from build123d import *

# Parameters (mm, degrees)
BOSS_EXTRU_1_DEPTH       = 15
ESQUISSE6_W              = 100
ESQUISSE6_H              = 15
ENL_V_MAT_EXTRU_1_DEPTH  = 215
ENL_V_MAT_EXTRU_10_REACH = 393.106
ESQUISSE11_R             = 2.25
ENL_V_MAT_EXTRU_11_REACH = 393.106
ESQUISSE8_R              = 2.25
CONG_10_R                = 10
CONG_11_R                = 2
ENL_V_MAT_EXTRU_12_REACH = 391.991


with BuildPart() as part:
    # Esquisse1 → Boss.-Extru.1 (new body)
    with BuildSketch(Plane(origin=(0, 0, 0), x_dir=(1, 0, 0), z_dir=(0, 1, 0))):
        Polygon((-76.643189126, -51.401333399), (63.356810874, 43.598666601), (163.356810874, 43.598666601), (303.356810874, -51.401333399), (303.356810874, -151.401333399), (163.356810874, -246.401333399), (63.356810874, -246.401333399), (-76.643189126, -151.401333399), align=None)
    extrude(amount=BOSS_EXTRU_1_DEPTH)

    # Esquisse6 → Enlèv. mat.-Extru.1 (cut)
    with BuildSketch(Plane.XY.offset(246.401333399)):
        with Locations((113.356810874, 7.5)):
            Rectangle(ESQUISSE6_W, ESQUISSE6_H)
    extrude(amount=-ENL_V_MAT_EXTRU_1_DEPTH, mode=Mode.SUBTRACT)

    # Esquisse11 → Enlèv. mat.-Extru.10 (cut, up to next)
    with BuildSketch(Plane(origin=(0, 15, 0), x_dir=(1, 0, 0), z_dir=(0, 1, 0)), mode=Mode.PRIVATE) as enl_v_mat_extru_10_sk1:
        with Locations(Location((53.356810874, -129.901333399, 0), (0, 0, 270))):
            Circle(ESQUISSE11_R)
    enl_v_mat_extru_10_tool1 = extrude(enl_v_mat_extru_10_sk1.sketch, amount=-ENL_V_MAT_EXTRU_10_REACH, mode=Mode.PRIVATE) & part.part
    # Esquisse11 → Enlèv. mat.-Extru.10 (cut, up to next)
    with BuildSketch(Plane(origin=(0, 15, 0), x_dir=(1, 0, 0), z_dir=(0, 1, 0)), mode=Mode.PRIVATE) as enl_v_mat_extru_10_sk2:
        with Locations(Location((53.356810874, -184.901333399, 0), (0, 0, 270))):
            Circle(ESQUISSE11_R)
    enl_v_mat_extru_10_tool2 = extrude(enl_v_mat_extru_10_sk2.sketch, amount=-ENL_V_MAT_EXTRU_10_REACH, mode=Mode.PRIVATE) & part.part
    # Esquisse11 → Enlèv. mat.-Extru.10 (cut, up to next)
    with BuildSketch(Plane(origin=(0, 15, 0), x_dir=(1, 0, 0), z_dir=(0, 1, 0)), mode=Mode.PRIVATE) as enl_v_mat_extru_10_sk3:
        with Locations(Location((173.356810874, -129.901333399, 0), (0, 0, 270))):
            Circle(ESQUISSE11_R)
    enl_v_mat_extru_10_tool3 = extrude(enl_v_mat_extru_10_sk3.sketch, amount=-ENL_V_MAT_EXTRU_10_REACH, mode=Mode.PRIVATE) & part.part
    # Esquisse11 → Enlèv. mat.-Extru.10 (cut, up to next)
    with BuildSketch(Plane(origin=(0, 15, 0), x_dir=(1, 0, 0), z_dir=(0, 1, 0)), mode=Mode.PRIVATE) as enl_v_mat_extru_10_sk4:
        with Locations(Location((173.356810874, -184.901333399, 0), (0, 0, 270))):
            Circle(ESQUISSE11_R)
    enl_v_mat_extru_10_tool4 = extrude(enl_v_mat_extru_10_sk4.sketch, amount=-ENL_V_MAT_EXTRU_10_REACH, mode=Mode.PRIVATE) & part.part
    add(enl_v_mat_extru_10_tool1.solids().sort_by_distance((53.356811, 15, 129.901333))[0], mode=Mode.SUBTRACT)
    add(enl_v_mat_extru_10_tool2.solids().sort_by_distance((53.356811, 15, 184.901333))[0], mode=Mode.SUBTRACT)
    add(enl_v_mat_extru_10_tool3.solids().sort_by_distance((173.356811, 15, 129.901333))[0], mode=Mode.SUBTRACT)
    add(enl_v_mat_extru_10_tool4.solids().sort_by_distance((173.356811, 15, 184.901333))[0], mode=Mode.SUBTRACT)

    # Esquisse8 → Enlèv. mat.-Extru.11 (cut, up to next)
    with BuildSketch(Plane(origin=(0, 15, 0), x_dir=(1, 0, 0), z_dir=(0, 1, 0)), mode=Mode.PRIVATE) as enl_v_mat_extru_11_sk1:
        with Locations(Location((180.356810874, -120.901333399, 0), (0, 0, 270))):
            Circle(ESQUISSE8_R)
    enl_v_mat_extru_11_tool1 = extrude(enl_v_mat_extru_11_sk1.sketch, amount=-ENL_V_MAT_EXTRU_11_REACH, mode=Mode.PRIVATE) & part.part
    # Esquisse8 → Enlèv. mat.-Extru.11 (cut, up to next)
    with BuildSketch(Plane(origin=(0, 15, 0), x_dir=(1, 0, 0), z_dir=(0, 1, 0)), mode=Mode.PRIVATE) as enl_v_mat_extru_11_sk2:
        with Locations(Location((180.356810874, -81.901333399, 0), (0, 0, 270))):
            Circle(ESQUISSE8_R)
    enl_v_mat_extru_11_tool2 = extrude(enl_v_mat_extru_11_sk2.sketch, amount=-ENL_V_MAT_EXTRU_11_REACH, mode=Mode.PRIVATE) & part.part
    # Esquisse8 → Enlèv. mat.-Extru.11 (cut, up to next)
    with BuildSketch(Plane(origin=(0, 15, 0), x_dir=(1, 0, 0), z_dir=(0, 1, 0)), mode=Mode.PRIVATE) as enl_v_mat_extru_11_sk3:
        with Locations(Location((46.356810874, -120.901333399, 0), (0, 0, 270))):
            Circle(ESQUISSE8_R)
    enl_v_mat_extru_11_tool3 = extrude(enl_v_mat_extru_11_sk3.sketch, amount=-ENL_V_MAT_EXTRU_11_REACH, mode=Mode.PRIVATE) & part.part
    # Esquisse8 → Enlèv. mat.-Extru.11 (cut, up to next)
    with BuildSketch(Plane(origin=(0, 15, 0), x_dir=(1, 0, 0), z_dir=(0, 1, 0)), mode=Mode.PRIVATE) as enl_v_mat_extru_11_sk4:
        with Locations(Location((46.356810874, -81.901333399, 0), (0, 0, 270))):
            Circle(ESQUISSE8_R)
    enl_v_mat_extru_11_tool4 = extrude(enl_v_mat_extru_11_sk4.sketch, amount=-ENL_V_MAT_EXTRU_11_REACH, mode=Mode.PRIVATE) & part.part
    add(enl_v_mat_extru_11_tool1.solids().sort_by_distance((180.356811, 15, 120.901333))[0], mode=Mode.SUBTRACT)
    add(enl_v_mat_extru_11_tool2.solids().sort_by_distance((180.356811, 15, 81.901333))[0], mode=Mode.SUBTRACT)
    add(enl_v_mat_extru_11_tool3.solids().sort_by_distance((46.356811, 15, 120.901333))[0], mode=Mode.SUBTRACT)
    add(enl_v_mat_extru_11_tool4.solids().sort_by_distance((46.356811, 15, 81.901333))[0], mode=Mode.SUBTRACT)

    # Congé10
    cong_10_edges = [part.edges().sort_by_distance(p)[0] for p in [
        (-76.643189126, 7.5, 51.401333399),
        (63.356810874, 7.5, -43.598666601),
        (163.356810874, 7.5, -43.598666601),
        (303.356810874, 7.5, 51.401333399),
        (303.356810874, 7.5, 151.401333399),
        (-76.643189126, 7.5, 151.401333399),
        (63.356810874, 7.5, 31.401333399),
        (163.356810874, 7.5, 31.401333399),
    ]]
    fillet(cong_10_edges, radius=CONG_10_R)

    # Congé11
    cong_11_edges = [part.edges().sort_by_distance(p)[0] for p in [
        (163.356810874, 7.5, 246.401333399),
        (63.356810874, 7.5, 246.401333399),
    ]]
    fillet(cong_11_edges, radius=CONG_11_R)

    # Esquisse12 → Enlèv. mat.-Extru.12 (cut, up to next)
    with BuildSketch(Plane(origin=(0, 15, 0), x_dir=(1, 0, 0), z_dir=(0, 1, 0)), mode=Mode.PRIVATE) as enl_v_mat_extru_12_sk1:
        with BuildLine():
            Line((46.009256573, -55.538188752), (18.058498347, -78.315798735))
            ThreePointArc((18.058498347, -78.315798735), (14.643777091, -83.767882822), (15.256670784, -90.171780344))
            Line((15.256670784, -90.171780344), (27.943631129, -118.361875593))
            ThreePointArc((27.943631129, -118.361875593), (31.633138728, -122.655474578), (37.06267458, -124.257847507))
            Line((37.06267458, -124.257847507), (53.356810874, -124.257847507))
            ThreePointArc((53.356810874, -124.257847507), (57.183645198, -123.496642832), (60.427878686, -121.328915318))
            Line((60.427878686, -121.328915318), (63.356810874, -118.39998313))
            Line((63.356810874, -118.39998313), (63.356810874, -59.592280682))
            Line((63.356810874, -59.592280682), (59.121809419, -54.561118788))
            ThreePointArc((59.121809419, -54.561118788), (52.42687157, -53.188778562), (46.009256573, -55.538188752))
        make_face()
    enl_v_mat_extru_12_tool1 = extrude(enl_v_mat_extru_12_sk1.sketch, amount=-ENL_V_MAT_EXTRU_12_REACH, mode=Mode.PRIVATE) & part.part
    # Esquisse12 → Enlèv. mat.-Extru.12 (cut, up to next)
    with BuildSketch(Plane(origin=(0, 15, 0), x_dir=(1, 0, 0), z_dir=(0, 1, 0)), mode=Mode.PRIVATE) as enl_v_mat_extru_12_sk2:
        with BuildLine():
            Line((166.285743062, -121.328915318), (163.356810874, -118.39998313))
            Line((163.356810874, -118.39998313), (163.356810874, -73.642376596))
            Line((163.356810874, -73.642376596), (176.462200108, -67.250451181))
            ThreePointArc((176.462200108, -67.250451181), (187.921289626, -66.549583242), (196.519678004, -74.156794674))
            Line((196.519678004, -74.156794674), (206.924784537, -95.490424571))
            ThreePointArc((206.924784537, -95.490424571), (205.909865534, -114.856232791), (188.948903611, -124.257847507))
            Line((188.948903611, -124.257847507), (173.356810874, -124.257847507))
            ThreePointArc((173.356810874, -124.257847507), (169.529976551, -123.496642832), (166.285743062, -121.328915318))
        make_face()
    enl_v_mat_extru_12_tool2 = extrude(enl_v_mat_extru_12_sk2.sketch, amount=-ENL_V_MAT_EXTRU_12_REACH, mode=Mode.PRIVATE) & part.part
    add(enl_v_mat_extru_12_tool1.solids().sort_by_distance((43.070441, 15, 90.852572))[0], mode=Mode.SUBTRACT)
    add(enl_v_mat_extru_12_tool2.solids().sort_by_distance((183.873626, 15, 97.045657))[0], mode=Mode.SUBTRACT)


solid = part.part
Could you check a few things on this model? Use its own coordinates, in mm. A direction names the side the tool comes from. Round coordinates to 2 decimals unless told otherwise and drop trailing zeros. Write each loop counter-clockwise with the first axis right and the second up, starting at its lowest first coordinate (ties: lowest second). Pieces come first, ordered by that corner, then holes. Notation, with made-up numbers: (6.25, 69.5) -> (21.25, 69.5) arc R14 cw to (21.25, 87.5) -> close; hole circle Ø2 at (0.25, 9.25). An arc over 180 degrees is marked (long way). Use a Markdown table: item, result.
1. For pin 1 Ø6 at (x, y) = (248, 13.5) entering from -Z; pin 2 Ø7.5 at (y, z) = (5, 161) entering from +X; pin 3 Ø3.5 at (x, z) = (53.36, 184.9) entering from +Y; pin 4 Ø7.5 at (x, y) = (116.5, 6.5) entering from +Z, each with a flat end and sliding along its axis, tell me the tip position at first contact or that it passes through.
Answer key:
| item | result |
|---|---|
| pin 1 | stops at z = 11.8 |
| pin 2 | stops at x = 294.74 |
| pin 3 | passes through |
| pin 4 | stops at z = 31.4 |
2. If we section it at D-D (x = -36): List the corners of the cut face in (y, z) for me.
Answer key:
| item | result |
|---|---|
| outline | (0, 23.82) -> (15, 23.82) -> (15, 178.98) -> (0, 178.98) -> close |
3. Please list where these lines run through material, in increasing order: probe 1 along X at (y, z) = (12.5, 135); probe 2 along X at (y, z) = (8.25, 69); probe 3 along X at (y, z) = (1.75, 58.5).
Answer key:
| item | result |
|---|---|
| probe 1 | x = -76.64 to 63.36, 163.36 to 303.36 |
| probe 2 | x = -76.64 to 29.49, 163.36 to 172.88, 192.38 to 303.36 |
| probe 3 | x = -76.64 to 42.37, 62.44 to 63.36, 163.36 to 303.36 |
4. Which directions (+Z, -Z, +X, -X, +Y, -Y) give clear straight access to the entire face, cutting with the end or side of a thin tool? Please do faces 4 (the face through (187.77, 7.6, 66.5)), 5 (the face through (-76.643, 7, 102)), 6 (the face through (63.357, 7, 181)).
Answer key:
| item | result |
|---|---|
| face 4 | +Y, -Y |
| face 5 | +Z, -Z, -X, +Y, -Y |
| face 6 | +Z, +Y, -Y |
5. We'd pull the mould along Z, two halves only. Please class faces 1 (the face through (160.35, 7.605, 34.253)), 2 (the face through (113, 7, -43.599)), 3 (the face through (181, 8, 124.258)): +Z half, -Z half, draft (parallel to the pull), parting line (faces both ways), or undercut.
Answer key:
| item | result |
|---|---|
| face 1 | +Z half |
| face 2 | -Z half |
| face 3 | undercut |
6. If we section it at C-C (y = 12.25): State how many separate pieces and enclosed holes the cut face has, then the cut area to 3 significant figures.
Answer key:
| item | result |
|---|---|
| separate pieces | 1 |
| enclosed holes | 4 |
| area | 57,200 mm^2 |
7. If we section it at A-A (x = 41): List the corners of the cut face in (y, z) for me, then the cut area to 3 significant figures.
Answer key:
| item | result |
|---|---|
| outline | (0, -28.43) -> (15, -28.43) -> (15, 59.62) -> (0, 59.62) -> close; (0, 124.26) -> (15, 124.26) -> (15, 231.23) -> (0, 231.23) -> close |
| area | 2,930 mm^2 |
8. If we section it at B-B (z = 224): List the corners of the cut face in (x, y) for me.
Answer key:
| item | result |
|---|---|
| outline | (30.34, 0) -> (63.36, 0) -> (63.36, 15) -> (30.34, 15) -> close; (163.36, 0) -> (196.37, 0) -> (196.37, 15) -> (163.36, 15) -> close |
